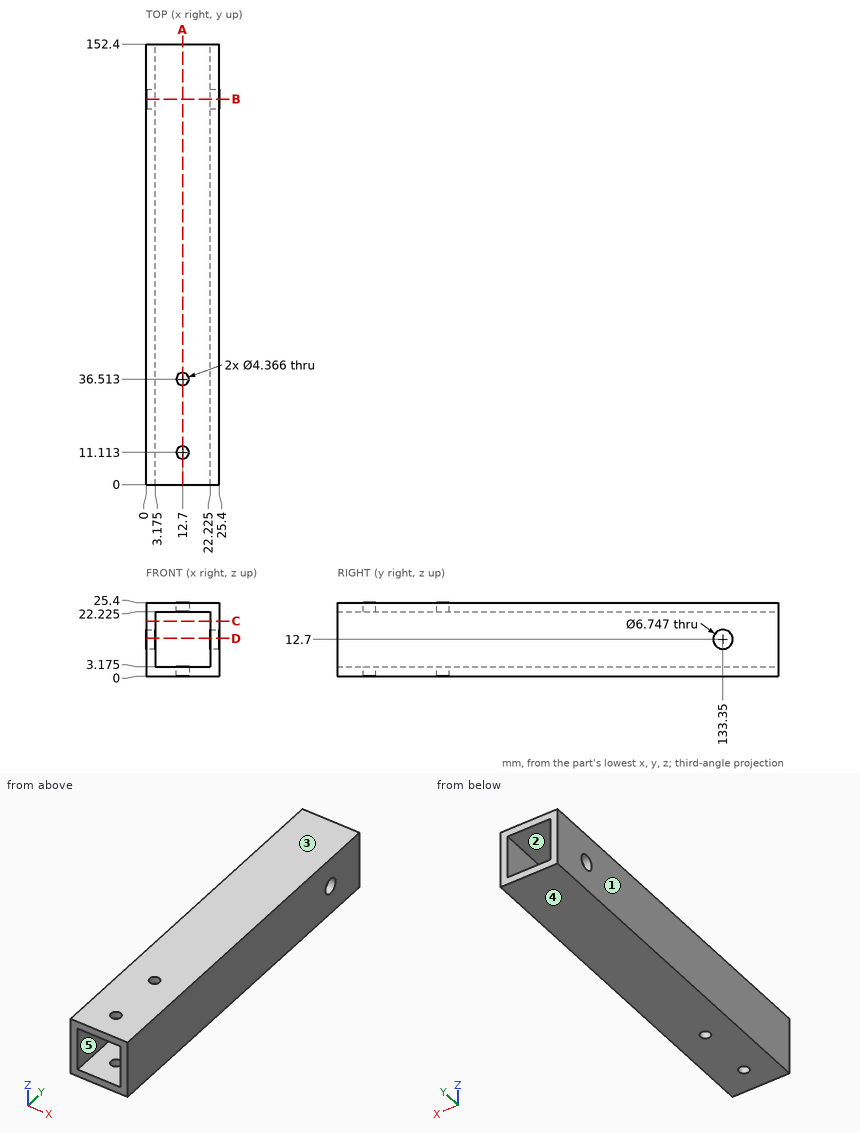
Geometry check sheet. Reference: drawing and pictorial views, mm from the part's lowest x, y, z. A direction names the side the tool comes from. Round coordinates to 2 decimals unless told otherwise and drop trailing zeros. Order: outer loops, then holes, each group sorted by start corner. A loop starts at its lowest first (then second) coordinate and runs counter-clockwise, first axis right, second up. Notation, with made-up numbers: (42.5, 0) - (61.5, 0) arc R16 cw to (61.5, 29) - close; hole circle Ø7 at (4.5, -2.5). An arc over 180 degrees is marked (long way). Write item = value, one per line.
Q1. Section check C-C (z = 19). Record the boundary of the cut face in (x, y) (1 decimal).
Computed:
outline = (0, 0) - (3.2, 0) - (3.2, 152.4) - (0, 152.4) - close; (22.2, 0) - (25.4, 0) - (25.4, 152.4) - (22.2, 152.4) - close
Q2. Draft check along Z on the marked faces 3, 4 and 5. Enter one of: pulls with the +Z half, pulls with the -Z half, needs draft (parallel to the pull), parting line crosses it, or undercut.
Computed:
face_3 = pulls with the +Z half
face_4 = pulls with the -Z half
face_5 = undercut
Q3. Section check D-D (z = 13). Record the boundary of the cut face in (x, y) (1 decimal).
Computed:
outline = (0, 0) - (3.2, 0) - (3.2, 130) - (0, 130) - close; (0, 136.7) - (3.2, 136.7) - (3.2, 152.4) - (0, 152.4) - close; (22.2, 0) - (25.4, 0) - (25.4, 130) - (22.2, 130) - close; (22.2, 136.7) - (25.4, 136.7) - (25.4, 152.4) - (22.2, 152.4) - close
Q4. Section check A-A (x = 12.7). Record the boundary of the cut face in (y, z) (1 decimal).
Computed:
outline = (0, 0) - (8.9, 0) - (8.9, 3.2) - (0, 3.2) - close; (0, 22.2) - (8.9, 22.2) - (8.9, 25.4) - (0, 25.4) - close; (13.3, 0) - (34.3, 0) - (34.3, 3.2) - (13.3, 3.2) - close; (13.3, 22.2) - (34.3, 22.2) - (34.3, 25.4) - (13.3, 25.4) - close; (38.7, 0) - (152.4, 0) - (152.4, 3.2) - (38.7, 3.2) - close; (38.7, 22.2) - (152.4, 22.2) - (152.4, 25.4) - (38.7, 25.4) - close
Q5. Thickness scan on line 1 along Y through (x, z) = (12.7, 23.65) (1 decimal); line 2 along Z through (x, y) = (6.25, 30) (1 decimal). Record the ranges inside material, lowest first.
Computed:
line_1 = 0 to 8.9, 13.3 to 34.3, 38.7 to 152.4
line_2 = 0 to 3.2, 22.2 to 25.4
Q6. Section check B-B (y = 133.35). Record the boundary of the cut face in (x, z) (1 decimal).
Computed:
outline = (0, 0) - (25.4, 0) - (25.4, 9.3) - (22.2, 9.3) - (22.2, 3.2) - (3.2, 3.2) - (3.2, 9.3) - (0, 9.3) - close; (0, 16.1) - (3.2, 16.1) - (3.2, 22.2) - (22.2, 22.2) - (22.2, 16.1) - (25.4, 16.1) - (25.4, 25.4) - (0, 25.4) - close
Q7. Tool access check on the marked faces 1 and 2. Record the directions out of +Z, -Z, +X, -X, +Y, -Y that give a thin tool (end or side, any length) a straight path to the whole face; none if there is none.
Computed:
face_1 = +Z, -Z, -X, +Y, -Y
face_2 = +Y, -Y
